Here's how the part is built. I have some questions about the finished solid (model axes, mm). Round coordinates to 2 decimals unless told otherwise and drop trailing zeros. Order: outer loops, then holes, each group sorted by start corner. A loop starts at its lowest first (then second) coordinate and runs counter-clockwise, first axis right, second up. Notation, with made-up numbers: (89, -27.5) -> (141, -27.5) arc R29 cw to (141, 1.5) -> close; hole circle Ø4 at (-30, 11.25). An arc over 180 degrees is marked (long way). Use a Markdown table: item, result. Add a question column.
Autodesk Fusion 360 part; units mm, degrees
sketch "Esboço1" plane through (0, 0, 0) normal (0, 0, 1) x (1, 0, 0)
  line L0 (0, 0) -> (88, 0)
  line L1 (-2.5, 203) -> (0, 0)
  line L2 (90.5, 203) -> (88, 0)
  line L3 (44, 235) -> (90.5, 203)
  line L4 (44, 235) -> (-2.5, 203)
  line L5 (88.487, 201.9575) -> (86.0245, 2)
  line L6 (1.9755, 2) -> (86.0245, 2)
  line L7 (-0.487, 201.9575) -> (1.9755, 2)
  line L8 (44, 232.5722) -> (-0.487, 201.9575)
  line L9 (44, 232.5722) -> (88.487, 201.9575)
  dimension "d1" = 88
  dimension "d7" = -2
sketch "Esboço2" plane through (0, 0, 5) normal (0, 0, 1) x (-1, 0, 0)
  line L0 (-1.9755, -2) -> (0.487, -201.9575)
  line L1 (0.487, -201.9575) -> (-44, -232.5722)
  line L2 (-44, -232.5722) -> (-88.487, -201.9575)
  line L3 (-88.487, -201.9575) -> (-86.0245, -2)
  line L4 (-86.0245, -2) -> (-1.9755, -2)
  line L5 (-90.5, -203) -> (-44, -235)
  line L6 (-44, -235) -> (2.5, -203)
  line L7 (2.5, -203) -> (0, 0)
  line L8 (0, 0) -> (-88, 0)
  line L9 (-88, 0) -> (-90.5, -203)
  line L10 (-44, -228.9304) -> (-85.4675, -200.3937)
  line L11 (-85.4675, -200.3937) -> (-83.0612, -5)
  line L12 (-83.0612, -5) -> (-4.9388, -5)
  line L13 (-4.9388, -5) -> (-2.5325, -200.3937)
  line L14 (-2.5325, -200.3937) -> (-44, -228.9304)
  dimension "d10" = 3
sketch "Esboço3" plane through (0, 0, 5) normal (0, 0, 1) x (-1, 0, 0)
  line L0 (-4.9388, -5) -> (-2.5325, -200.3937)
  line L1 (-2.5325, -200.3937) -> (-44, -228.9304)
  line L2 (-44, -228.9304) -> (-85.4675, -200.3937)
  line L3 (-85.4675, -200.3937) -> (-83.0612, -5)
  line L4 (-83.0612, -5) -> (-4.9388, -5)
  line L5 (-4.0422, -199.6117) -> (-44, -227.1096)
  line L6 (-44, -227.1096) -> (-83.9578, -199.6117)
  line L7 (-83.9578, -199.6117) -> (-81.5796, -6.5)
  line L8 (-81.5796, -6.5) -> (-6.4204, -6.5)
  line L9 (-6.4204, -6.5) -> (-4.0422, -199.6117)
  line L10 (-86.0245, -2) -> (-88.487, -201.9575)
  line L11 (-88.487, -201.9575) -> (-44, -232.5722)
  line L12 (-44, -232.5722) -> (0.487, -201.9575)
  line L13 (0.487, -201.9575) -> (-1.9755, -2)
  line L14 (-1.9755, -2) -> (-86.0245, -2)
  dimension "d13" = 1.5
sketch "Esboço4" plane through (0, 0, 5) normal (0, 0, 1) x (-1, 0, 0)
  line L0 (-81.5796, -6.5) -> (-6.4204, -6.5)
  line L1 (-6.4204, -6.5) -> (-4.0422, -199.6117)
  line L2 (-4.0422, -199.6117) -> (-44, -227.1096)
  line L3 (-44, -227.1096) -> (-83.9578, -199.6117)
  line L4 (-83.9578, -199.6117) -> (-81.5796, -6.5)
  line L5 (-44, -233.1791) -> (0.9903, -202.2181)
  line L6 (0.9903, -202.2181) -> (-1.4816, -1.5)
  line L7 (-1.4816, -1.5) -> (-86.5184, -1.5)
  line L8 (-86.5184, -1.5) -> (-88.9903, -202.2181)
  line L9 (-88.9903, -202.2181) -> (-44, -233.1791)
  line L10 (-83.0612, -5) -> (-85.4675, -200.3937)
  line L11 (-85.4675, -200.3937) -> (-44, -228.9304)
  line L12 (-44, -228.9304) -> (-2.5325, -200.3937)
  line L13 (-2.5325, -200.3937) -> (-4.9388, -5)
  line L14 (-4.9388, -5) -> (-83.0612, -5)
sketch "Esboço5" plane through (86.4868, -1.0651, 0) normal (-0.9999, 0.0123, 0) x (-0.0123, -0.9999, 0)
  line L0 (-2.5653, 5) -> (-2.5653, 65)
  line L1 (-2.5653, 65) -> (-203.2986, 65)
  line L2 (-203.2986, 65) -> (-203.2986, 5)
  line L3 (-2.5653, 65) -> (-2.5653, 63)
  line L4 (-2.5653, 63) -> (-10.5653, 63)
  line L5 (-10.5653, 63) -> (-10.5653, 60)
  line L6 (-10.5653, 60) -> (-2.5653, 60)
  line L7 (-203.2986, 5) -> (-2.5653, 5)
  dimension "d19" = 2
  dimension "d20" = 8
  dimension "d21" = 3
sketch "Esboço6" plane through (0, 0, 63) normal (0, 0, 1) x (-1, 0, 0)
  line L0 (-86.6169, -9.4994) -> (-78.6175, -9.5979)
  line L1 (-78.6175, -9.5979) -> (-78.519, -1.5985)
  line L2 (-78.519, -1.5985) -> (-86.5184, -1.5)
  line L3 (-78.519, -1.5985) -> (-86.6169, -9.4994)
  line L4 (-86.5184, -1.5) -> (-86.6169, -9.4994)
sketch "Esboço7" plane through (0, 0, 63) normal (0, 0, 1) x (-1, 0, 0)
  line L0 (-86.6169, -9.4994) -> (-78.519, -1.5985)
  line L1 (-78.519, -1.5985) -> (-86.5184, -1.5)
  circle A0 centre (-84.5431, -3.5245) radius 1
  line L2 (-86.5184, -1.5) -> (-86.6169, -9.4994)
  dimension "d26" = 2
sketch "Esboço8" plane through (1.4999, 0.0185, 0) normal (0.9999, 0.0123, 0) x (-0.0123, 0.9999, 0)
  line L0 (202.215, 5) -> (202.215, 65)
  line L1 (202.215, 65) -> (1.4816, 65)
  line L2 (1.4816, 65) -> (1.4816, 5)
  line L3 (1.4816, 65) -> (1.4816, 63)
  line L4 (1.4816, 63) -> (9.4816, 63)
  line L5 (9.4816, 63) -> (9.4816, 60)
  line L6 (9.4816, 60) -> (1.4816, 60)
  line L7 (1.4816, 5) -> (202.215, 5)
  dimension "d29" = 2
  dimension "d30" = 8
sketch "Esboço9" plane through (0, 0, 63) normal (0, 0, 1) x (-1, 0, 0)
  line L0 (-1.4816, -1.5) -> (-9.481, -1.5985)
  line L1 (-9.481, -1.5985) -> (-9.3825, -9.5979)
  line L2 (-9.3825, -9.5979) -> (-1.3831, -9.4994)
  line L3 (-9.481, -1.5985) -> (-1.3831, -9.4994)
  line L4 (-1.3831, -9.4994) -> (-1.4816, -1.5)
sketch "Esboço10" plane through (0, 0, 63) normal (0, 0, 1) x (-1, 0, 0)
  line L0 (-9.481, -1.5985) -> (-1.3831, -9.4994)
  line L1 (-1.4816, -1.5) -> (-9.481, -1.5985)
  circle A0 centre (-3.4569, -3.5245) radius 1
  line L2 (-1.3831, -9.4994) -> (-1.4816, -1.5)
  dimension "d35" = 2
sketch "Esboço11" plane through (-94.7554, 137.6915, 0) normal (0.5669, -0.8238, 0) x (0.8238, 0.5669, 0)
  line L0 (168.4368, 5) -> (168.4368, 65)
  line L1 (168.4368, 65) -> (113.8226, 65)
  line L2 (113.8226, 65) -> (113.8226, 5)
  line L3 (113.8226, 5) -> (168.4368, 5)
sketch "Esboço12" plane through (0, 0, 0) normal (0, 0, 1) x (1, 0, 0)
ref_plane "Plano de trabalho2" through (0, 0, 60) normal (0, 0, 1) x (1, 0, 0)
sketch "Esboço13" plane through (0, 0, 60) normal (0, 0, 1) x (1, 0, 0)
  line L0 (44, 229.2) -> (38, 229.2)
  line L1 (44, 229.2) -> (49.6973, 229.2)
  line L2 (38, 229.2) -> (44, 233.5)
  line L3 (44, 233.5) -> (49.6973, 229.2)
sketch "Esboço14" plane through (0, 0, 63) normal (0, 0, 1) x (-1, 0, 0)
  line L0 (-38, -229.2) -> (-49.6973, -229.2)
  line L1 (-49.6973, -229.2) -> (-44, -233.5)
  circle A0 centre (-43.9788, -231.1896) radius 1
  line L2 (-44, -233.5) -> (-38, -229.2)
  dimension "d48" = 2
sketch "Esboço15" plane through (0, 0, 65) normal (0, 0, 1) x (-1, 0, 0)
  line L0 (-44, -233.1791) -> (-88.9903, -202.2181)
  line L1 (-88.9903, -202.2181) -> (-86.5184, -1.5)
  line L2 (-86.5184, -1.5) -> (-1.4816, -1.5)
  line L3 (-1.4816, -1.5) -> (0.9903, -202.2181)
  line L4 (0.9903, -202.2181) -> (-44, -233.1791)
  line L5 (-88, 0) -> (-90.5, -203)
  line L6 (-90.5, -203) -> (-44, -235)
  line L7 (-44, -235) -> (2.5, -203)
  line L8 (2.5, -203) -> (0, 0)
  line L9 (0, 0) -> (-88, 0)
  line L10 (-196.5184, -1.5) -> (-111.4816, -1.5)
  line L11 (-198.9903, -202.2181) -> (-196.5184, -1.5)
  line L12 (-111.4816, -1.5) -> (-109.0097, -202.2181)
  line L13 (168.4368, 65) -> (113.8226, 65)
  line L14 (168.4368, 65) -> (113.8226, 65)
  line L15 (168.4368, 65) -> (113.8226, 65)
  line L16 (-154, -233.1791) -> (-198.9903, -202.2181)
  line L17 (-109.0097, -202.2181) -> (-154, -233.1791)
sketch "Esboço16" plane through (0, 0, 63) normal (0, 0, 1) x (-1, 0, 0)
  line L0 (-38, -229.2) -> (-49.6973, -229.2)
  line L1 (-49.6973, -229.2) -> (-44, -233.5)
  line L2 (-44, -233.5) -> (-38, -229.2)
sketch "Esboço17" plane through (0, 0, 67) normal (0, 0, 1) x (-1, 0, 0)
  line L0 (-109.0097, -202.2181) -> (-111.4816, -1.5)
  line L1 (-111.4816, -1.5) -> (-196.5184, -1.5)
  line L2 (-196.5184, -1.5) -> (-198.9903, -202.2181)
  line L3 (-198.9903, -202.2181) -> (-154, -233.1791)
  line L4 (-154, -233.1791) -> (-109.0097, -202.2181)
  circle A0 centre (-154, -231.1891) radius 1
  dimension "d55" = 1.99
  dimension "d56" = 2
sketch "Esboço18" plane through (0, 0, 63) normal (0, 0, 1) x (-1, 0, 0)
  circle A0 centre (-84.5431, -3.5245) radius 1
  line L0 (-86.6169, -9.4994) -> (-78.519, -1.5985)
  line L1 (-78.519, -1.5985) -> (-86.5184, -1.5)
  line L2 (-86.5184, -1.5) -> (-86.6169, -9.4994)
sketch "Esboço19" plane through (0, 0, 67) normal (0, 0, 1) x (-1, 0, 0)
  circle A0 centre (-154, -231.1891) radius 1
  line L0 (-109.0097, -202.2181) -> (-111.4816, -1.5)
  line L1 (-111.4816, -1.5) -> (-196.5184, -1.5)
  line L2 (-196.5184, -1.5) -> (-198.9903, -202.2181)
  line L3 (-198.9903, -202.2181) -> (-154, -233.1791)
  line L4 (-154, -233.1791) -> (-109.0097, -202.2181)
  circle A1 centre (-194.2131, -3.138) radius 1
  circle A2 centre (-113.2857, -2.8975) radius 1
  dimension "d59" = 2.828
  dimension "d60" = 2
  dimension "d61" = 2.282
  dimension "d62" = 2
sketch "Esboço20" plane through (0, 0, 65) normal (0, 0, 1) x (-1, 0, 0)
  line L0 (-44, -233.1791) -> (-88.9903, -202.2181)
  line L1 (-88.9903, -202.2181) -> (-86.5184, -1.5)
  line L2 (-86.5184, -1.5) -> (-1.4816, -1.5)
  line L3 (-1.4816, -1.5) -> (0.9903, -202.2181)
  line L4 (0.9903, -202.2181) -> (-44, -233.1791)
  line L5 (-88, 0) -> (-90.5, -203)
  line L6 (-90.5, -203) -> (-44, -235)
  line L7 (-44, -235) -> (2.5, -203)
  line L8 (2.5, -203) -> (0, 0)
  line L9 (0, 0) -> (-88, 0)
  line L10 (-44, -235) -> (2.5, -203)
  line L11 (-90.5, -203) -> (-90.8694, -232.9977)
  line L12 (-90.8694, -232.9977) -> (-44, -265)
  line L13 (2.5, -203) -> (2.8694, -232.9977)
  line L14 (2.8694, -232.9977) -> (-44, -265)
  line L15 (-90.5, -203) -> (-44, -235)
  dimension "d65" = 30
  dimension "d66" = 30
  dimension "d67" = 30
extrude "Extrusão17" add sketch "Esboço20" against normal blind 2 contours L6 L7 L10 L11 L12 L13 L14 L15
(1) I want a section at B-B on z = 64.5. List the corners of the cut face in (x, y) for me, and give its area (3 significant figures).
(2) If we mould it in two halves opening along X, with no side actions, what happens to faces 1 (the flat face through (67.575, 218.776, 64.014)), 2 (the flat face through (45, 240, 63)), 3 (the flat face through (21.075, 219.224, 64.014)), 4 (the flat face through (67.763, 248.775, 64.014))? For each: pulls with the +X half, pulls with the -X half, needs draft (parallel to the pull), parting line crosses it, or undercut.
(3) I'm going to push flat-ended pins straight in: P1, Ø1, axis at x = 73, z = 64, coming from the -Y side; P2, Ø12, axis at x = 73.5, y = 213.5, coming from the +Z side; P3, Ø1, axis at y = 235.5, z = 64, coming from the -X side. Where does each tip first touch, or does it pass through?
(4) I want a section at D-D on x = 78.5. List the corners of the cut face in (y, z) for me, and give its area (3 significant figures).
(5) I want a section at A-A on y = 212. List the corners of the cut face in (x, z) for me.
(6) Please list where these lines run through material, in increasing order: probe 1 along X at (y, z) = (233, 63.3); probe 2 along X at (y, z) = (226, 63.9); probe 3 along X at (y, z) = (241, 63.4). Write a range as from..to.
(7) I want a section at C-C on y = 219.5. List the corners of the cut face in (x, z) for me, and give its area (3 significant figures).
Output:
| question | item | result |
|---|---|---|
| 1 | outline | (-2.87, 233) -> (-2.5, 203) -> (44, 235) -> (90.5, 203) -> (90.87, 233) -> (44, 265) -> close |
| 1 | area | 2,810 mm² |
| 2 | face 1 | undercut |
| 2 | face 2 | needs draft |
| 2 | face 3 | undercut |
| 2 | face 4 | pulls with the +X half |
| 3 | P1 | y = 214.7 |
| 3 | P2 | z = 65 |
| 3 | P3 | x = 0.06 |
| 4 | outline | (211.26, 63) -> (241.44, 63) -> (241.44, 65) -> (211.26, 65) -> close |
| 4 | area | 60.4 mm² |
| 5 | outline | (-2.61, 63) -> (10.58, 63) -> (10.58, 65) -> (-2.61, 65) -> close; (77.42, 63) -> (90.61, 63) -> (90.61, 65) -> (77.42, 65) -> close |
| 6 | probe 1 | -2.87..41.09, 46.91..90.87 |
| 6 | probe 2 | -2.78..30.92, 57.08..90.78 |
| 6 | probe 3 | 8.85..79.15 |
| 7 | outline | (-2.7, 63) -> (21.48, 63) -> (21.48, 65) -> (-2.7, 65) -> close; (66.52, 63) -> (90.7, 63) -> (90.7, 65) -> (66.52, 65) -> close |
| 7 | area | 96.7 mm² |
